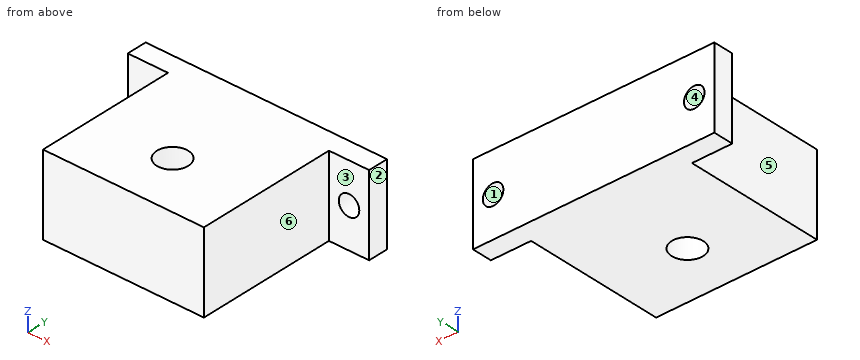
```python
from build123d import *

# Parameters (mm, degrees)
F1_DEPTH = 25.4
F4_R     = 3.2385
F5_DEPTH = 25.4
F3_R     = 3.2385
F6_DEPTH = 25.4
F7_R     = 4.953
F8_DEPTH = 25.4


with BuildPart() as f1:
    # F0 (on Top) → F1 (new body)
    with BuildSketch(Plane.XY):
        Polygon((76.2, 0), (0, 0), (0, -6.35), (12.703011, -6.35), (12.703011, -50.8), (63.5, -50.8), (63.5, -6.35), (76.2, -6.35), align=None)
    extrude(amount=F1_DEPTH)

    # F4 (on face) → F5 (cut)
    with BuildSketch(Plane.XZ.offset(6.35)):
        with Locations((6.35, 12.7)):
            Circle(F4_R)
    extrude(amount=-F5_DEPTH, mode=Mode.SUBTRACT)

    # F3 (on face) → F6 (cut)
    with BuildSketch(Plane.XZ.offset(6.35)):
        with Locations((69.85, 12.7)):
            Circle(F3_R)
    extrude(amount=-F6_DEPTH, mode=Mode.SUBTRACT)

    # F7 (on face) → F8 (cut)
    with BuildSketch(Plane.XY.offset(25.4)):
        with Locations((38.103011, -33.3375)):
            Circle(F7_R)
    extrude(amount=-F8_DEPTH, mode=Mode.SUBTRACT)


solid = f1.part
```
CAD build for the part. Positions are in the model's coordinates, mm. Face numbers are marked on the shaded views. A direction names the side the tool comes from. Give positions to 0.01 mm unless a question says otherwise; leave off trailing zeros. Write each loop counter-clockwise with the first axis right and the second up, starting at its lowest first coordinate (ties: lowest second). Pieces come first, ordered by that corner, then holes. Notation, with made-up numbers: M 57,1 L 79,1 A38 cw 79,40 Z; hole C -29,24.25 d10. An arc over 180 degrees is marked long. Return JSON: item names as keys, results as strings. Group by question number.
(1) 3-axis set-ups, long thin cutter, end or side, ignore diameter. For the marked faces 4, 5 and 6: which of +Z, -Z, +X, -X, +Y, -Y reach the whole face in a straight line?
(2) Flat gauge pins, fed straight in: pin 1 Ø4 at (x, z) = (6.35, 12.7) entering from +Y; pin 2 Ø1 at (y, z) = (-22, 18) entering from +X; pin 3 Ø10 at (x, z) = (6.5, 15.5) entering from -Y; pin 4 Ø12 at (y, z) = (-45.5, 22.5) entering from -X. Where does each tip first touch, or does it go through?
(3) Band-saw the part on A-A (z = 14.75). Give the cut face in (x, y), and give its area (3 significant figures).
(4) Band-saw the part on D-D (z = 20.75). Give the cut face in (x, y).
(5) Band-saw the part on C-C (y = -31). Give the cut face in (x, z), and give its area (3 significant figures).
(6) Band-saw the part on B-B (x = 6.35). Give the cut face in (y, z).
(7) Mould opens along X. For the marked faces 1, 2 and 3 say: pulls with the +X half, pulls with the -X half, needs draft (parallel to the pull), parting line crosses it, or undercut.
(8) Drill centre lines: L1, parallel to Z at x = 6, y = -1; L2, parallel to X at y = -27, z = 19; L3, parallel to Y at x = 8, z = 18.75. Where is each one in solid material? Low to high. Write a range as [from, to].
Entries:
{
 "1": {"face 4": "+Y, -Y", "face 5": "+Z, -Z, -X, -Y", "face 6": "+Z, -Z, +X, -Y"},
 "2": {"pin 1": "passes through", "pin 2": "stops at x = 63.5", "pin 3": "stops at y = -6.35", "pin 4": "stops at x = 12.7"},
 "3": {"outline": "M 0,-6.35 L 3.84,-6.35 L 3.84,0 L 0,0 Z; M 8.86,-6.35 L 12.7,-6.35 L 12.7,-50.8 L 63.5,-50.8 L 63.5,-6.35 L 67.34,-6.35 L 67.34,0 L 8.86,0 Z; M 72.36,-6.35 L 76.2,-6.35 L 76.2,0 L 72.36,0 Z; hole C 38.1,-33.34 d9.91", "area": "2,600 mm^2"},
 "4": {"outline": "M 0,-6.35 L 12.7,-6.35 L 12.7,-50.8 L 63.5,-50.8 L 63.5,-6.35 L 76.2,-6.35 L 76.2,0 L 0,0 Z; hole C 38.1,-33.34 d9.91"},
 "5": {"outline": "M 12.7,0 L 33.74,0 L 33.74,25.4 L 12.7,25.4 Z; M 42.47,0 L 63.5,0 L 63.5,25.4 L 42.47,25.4 Z", "area": "1,070 mm^2"},
 "6": {"outline": "M -6.35,0 L 0,0 L 0,9.46 L -6.35,9.46 Z; M -6.35,15.94 L 0,15.94 L 0,25.4 L -6.35,25.4 Z"},
 "7": {"face 1": "undercut", "face 2": "pulls with the +X half", "face 3": "needs draft"},
 "8": {"L1": "z = [0, 9.48], [15.92, 25.4]", "L2": "x = [12.7, 63.5]", "L3": "y = [-6.35, 0]"}
}
